The listing builds one solid part. Answer for the finished solid, in the listing's coordinates (mm). A direction names the side the tool comes from. Round coordinates to 2 decimals unless told otherwise and drop trailing zeros. Loops run counter-clockwise (first coordinate to the right, second up) from the corner with the lowest first, then second, coordinate; pieces in that order, holes last. Notation, with made-up numbers: M 59,8 L 92,8 A10 cw 92,26 Z; hole C 26.5,45 d6. An arc over 180 degrees is marked long. Put each result on its own line as item: value. Start each with the question number.
(1) Determine the mould class of faces 1 (the face through (5.99, 56.01, -45.61)), 2 (the face through (16.63, 20.11, -29.75)), 3 (the face through (20.2, 55, 37.3)) for opening direction Z: released by +Z, released by -Z, zero draft, split by the parting line, or undercut.
(2) Section B-B, the plane z = -35.5 is taken. Count the separate pieces of the cut face and the enclosed holes in it, then the cut area to 3 significant figures.
(3) Section A-A, the plane y = 27 is taken. Determine the outline of the cut face in (x, z).
(4) Which of the six approach directions +Z, -Z, +X, -X, +Y, -Y give full straight-line access (tool end or side, diameter ignored) to faces 4 (the face through (-8, 19, 25)), 5 (the face through (-14.284, 16.047, -41.055)), 6 (the face through (-20.2, 57, 37.3))?
(5) Straight lines are drawn through the part: line 1 (X direction, y = 27, z = 28.5); line 2 (X direction, y = 28, z = 0); line 3 (Z direction, x = 16, y = 29). For each, find the intervals that lie inside material, in ascending order.
(6) Flat-ended cylindrical pins translate along their axes: P1, Ø3, axis at y = 35, z = -29.5, coming from the -X side; P2, Ø4, axis at x = 21.5, y = 12.5, coming from the +Z side; P3, Ø11, axis at x = -5, y = 32.5, coming from the +Z side; P4, Ø20, axis at x = 0, y = 27, coming from the +Z side. Find the tip coordinate at first contact, or state that the pin passes through.
```python
from build123d import *

# Parameters (mm, degrees)
SKETCH19_R              = 11
CUT_EXTRUDE4_DEPTH      = 47
CUT_EXTRUDE4_DEPTH_BACK = 47
CUT_EXTRUDE5_START      = 38
SKETCH20_R              = 18
CUT_EXTRUDE5_DEPTH      = 51.0000001
BOSS_EXTRUDE2_START     = -37
SKETCH21_R              = 18
SKETCH21_R_2            = 11
BOSS_EXTRUDE2_DEPTH     = 12


with BuildPart() as part:
    # Sketch1 → Revolve1 (revolve)
    with BuildSketch(Plane.XY):
        with BuildLine():
            Line((-46, 0), (-46, 5))
            Line((-46, 5), (-42, 5))
            Line((-42, 5), (-42, 7))
            Line((-42, 7), (-46, 7))
            Line((-46, 7), (-46, 9))
            Line((-46, 9), (-46, 45))
            Line((-46, 45), (-46, 47))
            Line((-46, 47), (-42, 47))
            Line((-42, 47), (-42, 50))
            Line((-42, 50), (-46, 50))
            Line((-46, 50), (-46, 52))
            Line((-46, 52), (-42, 52))
            Line((-42, 52), (-42, 55))
            Line((-42, 55), (-46, 55))
            Line((-46, 55), (-46, 57))
            Line((-46, 57), (-42, 57))
            Line((-42, 57), (-42, 60))
            Line((-42, 60), (-46, 60))
            Line((-46, 60), (-46, 62))
            Line((-46, 62), (-42, 62))
            Line((-42, 62), (-42, 65))
            Line((-42, 65), (-46, 65))
            Line((-46, 65), (-46, 69))
            ThreePointArc((-46, 69), (-23.174880185, 73.257119382), (0, 74.683334091))
            Line((0, 74.683334091), (0, 69))
            Line((0, 69), (0, 60))
            Line((0, 60), (-37, 60))
            Line((-37, 60), (-37, 47))
            Line((-37, 47), (-37, 9))
            Line((-37, 9), (-37, 0))
            Line((-37, 0), (-46, 0))
        make_face()
    revolve(axis=Axis((0, 165.443928378, 0), (0, -1, 0)))

    # Sketch19 → Cut-Extrude4 (cut, two sides)
    with BuildSketch(Plane.XY) as cut_extrude4_sk:
        with Locations((0, 27)):
            Circle(SKETCH19_R)
    extrude(amount=CUT_EXTRUDE4_DEPTH, mode=Mode.SUBTRACT)
    extrude(cut_extrude4_sk.sketch, amount=-CUT_EXTRUDE4_DEPTH_BACK, mode=Mode.SUBTRACT)

    # Sketch20 → Cut-Extrude5 (cut)
    with BuildSketch(Plane.XY.offset(CUT_EXTRUDE5_START)):
        with Locations((0, 27)):
            Circle(SKETCH20_R)
    cut_extrude5 = extrude(amount=CUT_EXTRUDE5_DEPTH, mode=Mode.SUBTRACT)

    # Mirror1: Cut-Extrude5 across plane
    add(cut_extrude5.mirror(Plane.XY), mode=Mode.SUBTRACT)

    # Sketch21 → Boss-Extrude2 (add)
    with BuildSketch(Plane.XY.offset(BOSS_EXTRUDE2_START)):
        with Locations((0, 27)):
            Circle(SKETCH21_R)
        with Locations((0, 27)):
            Circle(SKETCH21_R_2, mode=Mode.SUBTRACT)
    boss_extrude2 = extrude(amount=BOSS_EXTRUDE2_DEPTH)

    # Mirror2: Boss-Extrude2 across plane
    add(boss_extrude2.mirror(Plane.XY))


solid = part.part
```
Recorded:
1. face 1: split by the parting line
1. face 2: undercut
1. face 3: zero draft
2. separate pieces: 1
2. enclosed holes: 2
2. area: 3,010 mm²
3. outline: M -18,-42.33 L -18,-38 L -11,-38 L -11,-25 L -18,-25 L -18,-32.33 A37 cw -18,32.33 L -18,25 L -11,25 L -11,38 L -18,38 L -18,42.33 A46 ccw Z; M 11,-38 L 18,-38 L 18,-42.33 A46 ccw 18,42.33 L 18,38 L 11,38 L 11,25 L 18,25 L 18,32.33 A37 cw 18,-32.33 L 18,-25 L 11,-25 Z
4. face 4: -Y
4. face 5: -Z
4. face 6: none
5. line 1: x = -36.11 to -23.6, -18 to -11, 11 to 18, 23.6 to 36.11
5. line 2: x = -46 to -37, 37 to 46
5. line 3: z = -38 to -25, 25 to 38
6. P1: stops at x = -36.5
6. P2: stops at z = 41.66
6. P3: stops at z = 38
6. P4: passes through
